Autodesk Inventor part; units mm, degrees
ref_plane "YZ Plane" through (0, 0, 0) normal (1, 0, 0) x (0, 1, 0)
ref_plane "XZ Plane" through (0, 0, 0) normal (0, 1, 0) x (-1, 0, 0)
ref_plane "XY Plane" through (0, 0, 0) normal (0, 0, 1) x (1, 0, 0)
sketch "Sketch1" plane through (0, 0, 0) normal (0, 1, 0) x (-1, 0, 0)
  circle A0 centre (0, 0) radius 14
  line L0 (13.2665, 20) -> (-13.2665, 20)
  line L1 (13.2665, -20) -> (-13.2665, -20)
  arc A1 (13.2665, -20) -> (13.2665, 20) centre (0, 0) ccw
  arc A2 (-13.2665, 20) -> (-13.2665, -20) centre (0, 0) ccw
  dimension "d1" = 28
  dimension "d2" = 20
  dimension "d3" = 20
  dimension "d19" = 24
extrude "Extrusion1" add sketch "Sketch1" along normal blind 10
sketch "Sketch2" plane through (0, 10, 0) normal (0, 1, 0) x (1, 0, 0)
  circle A0 centre (0, 0) radius 14
  line L0 (-13.2665, -20) -> (13.2665, -20)
  arc A1 (13.2665, -20) -> (13.2665, 20) centre (0, 0) ccw
  line L1 (13.2665, 20) -> (-13.2665, 20)
  arc A2 (-13.2665, 20) -> (-13.2665, -20) centre (0, 0) ccw
  circle A3 centre (-19, 0) radius 2.75
  circle A4 centre (-13.435, 13.435) radius 2.75
  circle A5 centre (-13.435, -13.435) radius 2.75
  line L2 (0, -20) -> (0, 20)
  line L3 (13.2665, 20) -> (-13.2665, 20)
  circle A6 centre (19, 0) radius 2.75
  circle A7 centre (13.435, 13.435) radius 2.75
  circle A8 centre (13.435, -13.435) radius 2.75
  dimension "d6" = 5.5
  dimension "d7" = 0
  dimension "d8" = 24
  dimension "d9" = 28
  dimension "d10" = 19
  dimension "d11" = 5.5
  dimension "d12" = 13.435
  dimension "d13" = 13.435
  dimension "d14" = 5.5
  dimension "d15" = 13.435
  dimension "d16" = 13.435
  dimension "d20" = 38
extrude "Extrusion2" cut sketch "Sketch2" against normal blind 10 contours A3 | A4 | A5 | A6 | A7 | A8
sketch "Sketch3" plane through (0, 10, 0) normal (0, 1, 0) x (1, 0, 0)
  circle A0 centre (0, 0) radius 14
  circle A1 centre (0, 0) radius 10
  dimension "d21" = 20
extrude "Extrusion3" add sketch "Sketch3" against normal blind 43
properties part number "PowerScrewNut"
Here's how the part is built. I have some questions about the finished solid (model axes, mm). A direction names the side the tool comes from. Coordinates: 2 decimals unless noted, no trailing zeros. Order: outer loops, then holes, each group sorted by start corner. A loop starts at its lowest first (then second) coordinate and runs counter-clockwise, first axis right, second up. Notation, with made-up numbers: (-17.5, 20) - (36.5, 20) arc R25 ccw to (36.5, 35) - close; hole circle Ø2 at (31.25, -26.75). An arc over 180 degrees is marked (long way). One line per question, with ' | ' between items.
(1) Suppose I cut it at C-C on z = -5. List the corners of the cut face in (x, y) for me, and give its area (3 significant figures).
Report:
outline: (-23.47, 0) - (-13.08, 0) - (-13.08, -33) - (-8.66, -33) - (-8.66, 10) - (-23.47, 10) - close; (8.66, -33) - (13.08, -33) - (13.08, 0) - (23.47, 0) - (23.47, 10) - (8.66, 10) - close | area: 588 mm2
(2) If I drill on L1, parallel to X at y = 5.5, z = 2.5; L2, parallel to Z at x = 0, y = -6; L3, parallel to Y at x = 15, z = 17, over which ranges is the centre line in solid material (lowest first)?
Report:
L1: x = -23.87 to -20.15, -17.85 to -9.68, 9.68 to 17.85, 20.15 to 23.87 | L2: z = -14 to -10, 10 to 14 | L3: y = 0 to 10
(3) If we mould it in two halves opening along Z, with no side actions, what happens to faces 3 (the flat face through (0, 5, -20)), 4 (the cylindrical face through (11.408, 5.07, -15.294)), 5 (the cylindrical face through (-16.182, 5.07, 13.314)), 6 (the cylindrical face through (12.932, -16.269, 5.362))? For each: pulls with the +Z half, pulls with the -Z half, needs draft (parallel to the pull), parting line crosses it, or undercut.
Report:
face 3: pulls with the -Z half | face 4: undercut | face 5: undercut | face 6: parting line crosses it
(4) Suppose I cut it at D-D on y = 1. State how many separate pieces and enclosed holes the cut face has, and give its area (3 significant figures).
Report:
separate pieces: 1 | enclosed holes: 7 | area: 1,210 mm2
(5) Suppose I cut it at B-B on z = 0. List the corners of the cut face in (x, y) for me.
Report:
outline: (-24, 0) - (-21.75, 0) - (-21.75, 10) - (-24, 10) - close; (-16.25, 0) - (-14, 0) - (-14, -33) - (-10, -33) - (-10, 10) - (-16.25, 10) - close; (10, -33) - (14, -33) - (14, 0) - (16.25, 0) - (16.25, 10) - (10, 10) - close; (21.75, 0) - (24, 0) - (24, 10) - (21.75, 10) - close
(6) Will these pins go through, and if not, where does the flat tip stop? pin 1 (1 mm diameter, centred on x = -9, z = 1, fed in from -Y); pin 2 (6 mm diameter, centred on x = -0.5, y = -10.5, fed in from +Z); pin 3 (1.5 mm diameter, centred on x = 7.5, y = -25.5, fed in from +Z); pin 4 (6.5 mm diameter, centred on x = -13.435, z = -13.435, fed in from -Y).
Report:
pin 1: passes through | pin 2: stops at z = 14 | pin 3: stops at z = 12.27 | pin 4: stops at y = 0
(7) For faces 1 (the flat face through (11, 0, 9)), 2 (the cylindrical face through (-21.747, 5.07, -0.121)), which set-ups out of +Z, -Z, +X, -X, +Y, -Y let a thin tool reach every point of the face, with its end or its side?
Report:
face 1: -Y | face 2: +Y, -Y
(8) Suppose I cut it at A-A on x = 0. List the corners of the cut face in (y, z) for me.
Report:
outline: (-33, -14) - (0, -14) - (0, -20) - (10, -20) - (10, -10) - (-33, -10) - close; (-33, 10) - (10, 10) - (10, 20) - (0, 20) - (0, 14) - (-33, 14) - close
